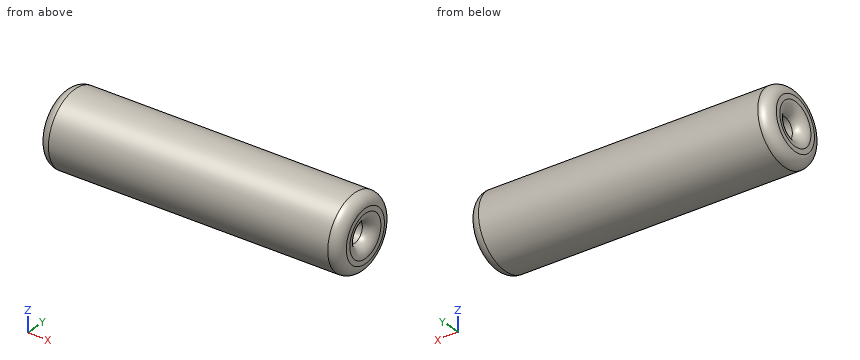
from build123d import *

# Parameters (mm, degrees)
F1_W = 140.3701454401
F1_H = 12.250483036
F5_R = 5
F6_R = 5


# Not quite as in the source:
# - a feature of the source that left no trace in its solid (it failed there, or was rolled back) is left out


with BuildPart() as f4:
    # F1 (on Front) → F4 (revolve)
    with BuildSketch(Plane.XZ):
        with Locations((270.1073512435, 393.0281996727)):
            Rectangle(F1_W, F1_H)
    revolve(axis=Axis((279.5873135328, 0, 382.010191679), (1, 0, 0)))

    # F5
    f5_edges = [f4.edges().sort_by_distance(p)[0] for p in [
        (340.292424, 0, 377.117425),
        (340.292424, 0, 364.866942),
    ]]
    fillet(f5_edges, radius=F5_R)

    # F6
    f6_edges = [f4.edges().sort_by_distance(p)[0] for p in [
        (199.922279, 0, 364.866942),
        (199.922279, 0, 377.117425),
    ]]
    fillet(f6_edges, radius=F6_R)


solid = f4.part
The listing builds one solid part. Answer for the finished solid, in the listing's coordinates (mm). Coordinates: 2 decimals unless noted, no trailing zeros. Write each loop counter-clockwise with the first axis right and the second up, starting at its lowest first coordinate (ties: lowest second). Pieces come first, ordered by that corner, then holes. Notation, with made-up numbers: M 41,10 L 70,10 A28 cw 70,34 Z; hole C 44.5,79.25 d4. An arc over 180 degrees is marked long. Use one line per item in the form item = value.
Item 1: Find section A-A, the plane y = 0. Give the vertices of the cut face in (x, z).
Model answer:
outline = M 199.92,369.87 A5 ccw 204.92,364.87 L 335.29,364.87 A5 ccw 340.29,369.87 L 340.29,372.12 A5 ccw 335.29,377.12 L 204.92,377.12 A5 ccw 199.92,372.12 Z; M 199.92,391.9 A5 ccw 204.92,386.9 L 335.29,386.9 A5 ccw 340.29,391.9 L 340.29,394.15 A5 ccw 335.29,399.15 L 204.92,399.15 A5 ccw 199.92,394.15 Z
Item 2: Given P1, Ø1, axis at x = 319.5, y = -13.5, coming from the +Z side; P2, Ø10, axis at y = -12, z = 394.5, coming from the -X side; P3, Ø3, axis at x = 227.5, z = 379.5, coming from the +Y side, each flat-ended and moving along its own axis, determine where each tip first touches the part or whether it passes through.
Model answer:
P1 = 393.19
P2 = 199.93
P3 = 17.11
Item 3: Find the intervals of material crossed by probe 1 along Z at (x, y) = (293, 0); probe 2 along Z at (x, y) = (286, -0.5); probe 3 along Y at (x, z) = (305.5, 382.5), in increasing order.
Model answer:
probe_1 = 364.87 to 377.12, 386.9 to 399.15
probe_2 = 364.87 to 377.14, 386.88 to 399.15
probe_3 = -17.14 to -4.87, 4.87 to 17.14
Item 4: Find section B-B, the plane x = 248. Give the vertices of the cut face in (y, z).
Model answer:
outline = C 0,382.01 d34.29; hole C 0,382.01 d9.79
